Source: CAD feature listing. Evaluate the final solid. Frame: model axes, mm. Face numbers are marked on the shaded views. Give positions to 0.01 mm unless a question says otherwise; leave off trailing zeros. Loops run counter-clockwise (first coordinate to the right, second up) from the corner with the lowest first, then second, coordinate; pieces in that order, holes last. Notation, with made-up numbers: (-39, -28.75) -> (-32, -28.75) arc R34 cw to (-32, 7.25) -> close; hole circle Ø10 at (40.25, 85). An arc over 180 degrees is marked (long way). Return JSON: item names as keys, results as strings. Group by question number.
(1) Draft query along X for the marked faces 1, 2 and 3. Return one class per face: released by +X, released by -X, zero draft, split by the parting line, or undercut.
(2) Cut plane B-B on y = 3.5. Return loops of the section in (x, z).
(3) Ray query, line 1 (Z direction, x = 9, y = 9.75); line 2 (X direction, y = 4, z = -4.5); line 3 (X direction, y = 1.5, z = -18). Return the intervals inside material, ascending. Write a range as from..to.
(4) Cut plane A-A on z = -5. Return loops of the section in (x, y), then the cut area to 3 significant figures.
(5) Cut plane C-C on z = -14. Return loops of the section in (x, y), then the cut area to 3 significant figures.
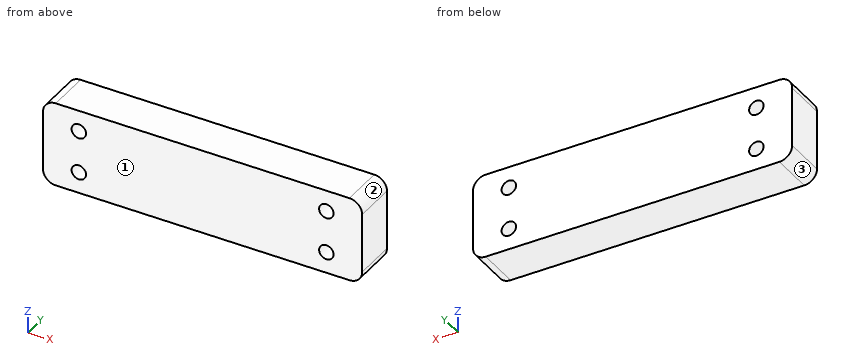
```python
from build123d import *

# Parameters (mm, degrees)
SKETCH1_W            = 75
SKETCH1_H            = 20
BOSS_EXTRUDE1_DEPTH  = 10
FILLET1_R            = 3
M3_CLEARANCE_HOLE1_D = 3.4


with BuildPart() as part:
    # Sketch1 → Boss-Extrude1 (new body)
    with BuildSketch(Plane(origin=(0, 0, 0), x_dir=(1, 0, 0), z_dir=(0, 1, 0))):
        with Locations((37.5, 10)):
            Rectangle(SKETCH1_W, SKETCH1_H)
    extrude(amount=BOSS_EXTRUDE1_DEPTH)

    # Fillet1
    fillet1_edges = [part.edges().sort_by_distance(p)[0] for p in [
        (0, 5, -20),
        (75, 5, -20),
        (75, 5, 0),
        (0, 5, 0),
    ]]
    fillet(fillet1_edges, radius=FILLET1_R)

    # M3 Clearance Hole1 (through all)
    with Locations(Plane(origin=(67.535318197, 10, -35.416339767), x_dir=(1, 0, 0), z_dir=(0, 1, 0))):
        with Locations((-0.954318197, -20.416339767), (-0.954318197, -30.416339767), (-59.116318197, -30.416339767), (-59.116318197, -20.416339767)):
            Hole(M3_CLEARANCE_HOLE1_D / 2)


solid = part.part
```
Answers:
{
 "1": {"face 1": "zero draft", "face 2": "released by +X", "face 3": "released by -X"},
 "2": {"outline": "(0, -17) arc R3 ccw to (3, -20) -> (72, -20) arc R3 ccw to (75, -17) -> (75, -3) arc R3 ccw to (72, 0) -> (3, 0) arc R3 ccw to (0, -3) -> close; hole circle Ø3.4 at (8.42, -15); hole circle Ø3.4 at (8.42, -5); hole circle Ø3.4 at (66.58, -15); hole circle Ø3.4 at (66.58, -5)"},
 "3": {"line 1": "-20..-16.6, -13.4..-6.6, -3.4..0", "line 2": "0..6.79, 10.04..64.96, 68.21..75", "line 3": "0.17..74.83"},
 "4": {"outline": "(0, 0) -> (6.72, 0) -> (6.72, 10) -> (0, 10) -> close; (10.12, 0) -> (64.88, 0) -> (64.88, 10) -> (10.12, 10) -> close; (68.28, 0) -> (75, 0) -> (75, 10) -> (68.28, 10) -> close", "area": "682 mm²"},
 "5": {"outline": "(0, 0) -> (7.04, 0) -> (7.04, 10) -> (0, 10) -> close; (9.79, 0) -> (65.21, 0) -> (65.21, 10) -> (9.79, 10) -> close; (67.96, 0) -> (75, 0) -> (75, 10) -> (67.96, 10) -> close", "area": "695 mm²"}
}
